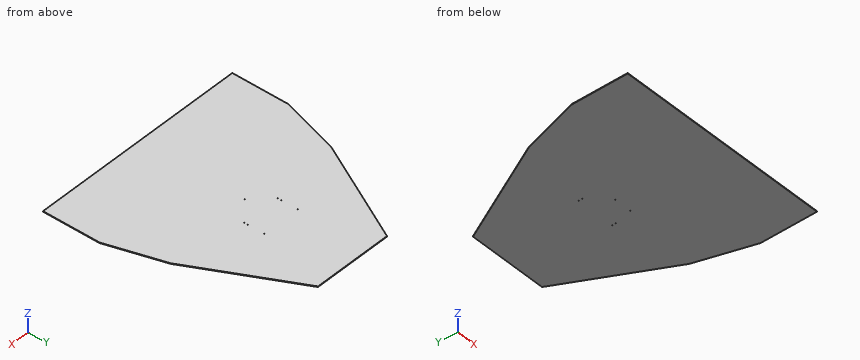
```python
from build123d import *

# Parameters (mm, degrees)
F0_R     = 2.05
F1_DEPTH = 5


with BuildPart() as f1:
    # F0 (on Top) → F1 (new body)
    with BuildSketch(Plane.XY):
        Polygon((-960, -460), (-960, -960), (960, -960), (960, -460), (812.5, 40), (555.555556, 540), (-555.555556, 540), (-812.5, 40), align=None)
        with Locations((-132.5, -28.5)):
            Circle(F0_R, mode=Mode.SUBTRACT)
        with Locations((-17.5, -28.5)):
            Circle(F0_R, mode=Mode.SUBTRACT)
        with Locations((132.5, -28.5)):
            Circle(F0_R, mode=Mode.SUBTRACT)
        with Locations((-170, 130.5)):
            Circle(F0_R, mode=Mode.SUBTRACT)
        with Locations((-170, 160.5)):
            Circle(F0_R, mode=Mode.SUBTRACT)
        with Locations((-170, 278.5)):
            Circle(F0_R, mode=Mode.SUBTRACT)
        with Locations((-170, 308.5)):
            Circle(F0_R, mode=Mode.SUBTRACT)
        with Locations((170, 130.5)):
            Circle(F0_R, mode=Mode.SUBTRACT)
        with Locations((170, 160.5)):
            Circle(F0_R, mode=Mode.SUBTRACT)
        with Locations((170, 278.5)):
            Circle(F0_R, mode=Mode.SUBTRACT)
        with Locations((170, 308.5)):
            Circle(F0_R, mode=Mode.SUBTRACT)
        Polygon((-350, 940), (-555.555556, 540), (555.555556, 540), (350, 940), align=None)
    extrude(amount=-F1_DEPTH)


solid = f1.part
```
Could you check a few things on this model? Use its own coordinates, in mm. Round coordinates to 2 decimals unless told otherwise and drop trailing zeros. Write each loop counter-clockwise with the first axis right and the second up, starting at its lowest first coordinate (ties: lowest second). Pieces come first, ordered by that corner, then holes.
(1) Suppose I cut it at A-A on z = -3.35. State how many separate pieces and enclosed holes the cut face has, and give its area (3 significant figures).
Findings below:
separate pieces: 1
enclosed holes: 11
area: 2,890,000 mm2
(2) If I drill on probe 1 along Y at (x, z) = (-170, -3.25); probe 2 along X at (y, z) = (92, -1.85); probe 3 along X at (y, z) = (43.5, -1.25), over which ranges is the centre line in solid material (lowest first)?
Findings below:
probe 1: y = -960 to 128.45, 132.55 to 158.45, 162.55 to 276.45, 280.55 to 306.45, 310.55 to 940
probe 2: x = -785.78 to 785.78
probe 3: x = -810.7 to 810.7
(3) For pin 1 (2.5 mm diameter, centred on x = 170, y = 308.5, fed in from -Z); pin 2 (1 mm diameter, centred on y = 370.5, z = -2.5, fed in from -X), each with a flat end and sliding along its axis, tell me the tip position at first contact or that it passes through.
Findings below:
pin 1: passes through
pin 2: stops at x = -642.92
(4) Suppose I cut it at C-C on x = -745.5. Write out the boundary of the cut face in (y, z).
Findings below:
outline: (-960, -5) - (170.38, -5) - (170.38, 0) - (-960, 0) - close
(5) Suppose I cut it at B-B on y = -224. Write out the boundary of the cut face in (x, z), and give its area (3 significant figures).
Findings below:
outline: (-890.38, -5) - (890.38, -5) - (890.38, 0) - (-890.38, 0) - close
area: 8,900 mm2
